The model under review builds one solid part; all positions refer to its coordinate system, in mm. Face numbers are marked on the shaded views. A direction names the side the tool comes from. Round coordinates to 2 decimals unless told otherwise and drop trailing zeros. Order: outer loops, then holes, each group sorted by start corner. A loop starts at its lowest first (then second) coordinate and runs counter-clockwise, first axis right, second up.
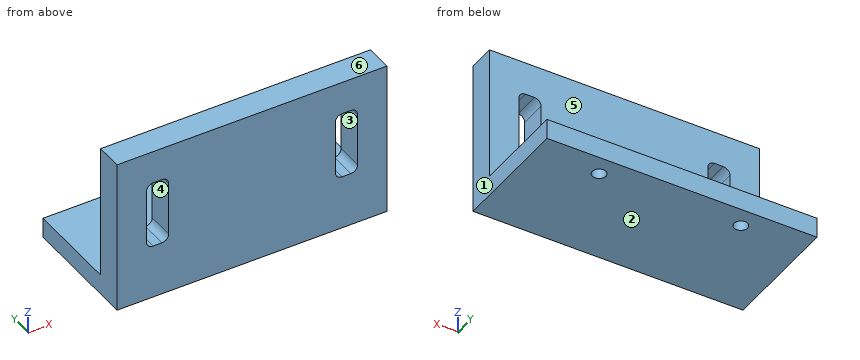
from build123d import *

# Parameters (mm, degrees)
SKETCH1_W           = 40
SKETCH1_H           = 20
BOSS_EXTRUDE1_DEPTH = 4
SKETCH2_W           = 40
SKETCH2_H           = 3
BOSS_EXTRUDE2_DEPTH = 18
SKETCH3_R           = 1
CUT_EXTRUDE1_DEPTH  = 36.397740041


with BuildPart() as part:
    # Sketch1 → Boss-Extrude1 (new body)
    with BuildSketch(Plane(origin=(0, 0, 0), x_dir=(1, 0, 0), z_dir=(0, 1, 0))):
        Rectangle(SKETCH1_W, SKETCH1_H)
        with BuildLine():
            Line((13.35, 4.93188921), (14.65, 4.93188921))
            ThreePointArc((14.65, 4.93188921), (15.357106781, 4.638995992), (15.65, 3.93188921))
            Line((15.65, 3.93188921), (15.65, -4.06811079))
            ThreePointArc((15.65, -4.06811079), (15.357106781, -4.775217571), (14.65, -5.06811079))
            Line((14.65, -5.06811079), (13.35, -5.06811079))
            ThreePointArc((13.35, -5.06811079), (12.642893219, -4.775217571), (12.35, -4.06811079))
            Line((12.35, -4.06811079), (12.35, 3.93188921))
            ThreePointArc((12.35, 3.93188921), (12.642893219, 4.638995992), (13.35, 4.93188921))
        make_face(mode=Mode.SUBTRACT)
        with BuildLine():
            Line((-15.65, 3.93188921), (-15.65, -4.06811079))
            ThreePointArc((-15.65, -4.06811079), (-15.357106781, -4.775217571), (-14.65, -5.06811079))
            Line((-14.65, -5.06811079), (-13.35, -5.06811079))
            ThreePointArc((-13.35, -5.06811079), (-12.642893219, -4.775217571), (-12.35, -4.06811079))
            Line((-12.35, -4.06811079), (-12.35, 3.93188921))
            ThreePointArc((-12.35, 3.93188921), (-12.642893219, 4.638995992), (-13.35, 4.93188921))
            Line((-13.35, 4.93188921), (-14.65, 4.93188921))
            ThreePointArc((-14.65, 4.93188921), (-15.357106781, 4.638995992), (-15.65, 3.93188921))
        make_face(mode=Mode.SUBTRACT)
    extrude(amount=BOSS_EXTRUDE1_DEPTH)

    # Sketch2 → Boss-Extrude2 (add)
    with BuildSketch(Plane(origin=(0, 0, 0), x_dir=(1, 0, 0), z_dir=(0, 1, 0))):
        with Locations((0, 11.5)):
            Rectangle(SKETCH2_W, SKETCH2_H)
    extrude(amount=BOSS_EXTRUDE2_DEPTH)

    # Sketch3 → Cut-Extrude1 (cut, through all)
    with BuildSketch(Plane(origin=(0, 0, -13), x_dir=(-1, 0, 0), z_dir=(0, 0, -1))):
        with Locations((10.5, 15.063230043)):
            Circle(SKETCH3_R)
        with Locations((-10.5, 15.063230043)):
            Circle(SKETCH3_R)
    extrude(amount=-CUT_EXTRUDE1_DEPTH, mode=Mode.SUBTRACT)


solid = part.part
(1) We need section A-A (z = 2.75). Give the boundary of the cut face in (x, y), and give its area (3 significant figures).
(2) We need section C-C (y = 1.5). Give the boundary of the cut face in (x, z).
(3) To check wall thickness, follow L1, parallel to X at y = 1, z = 3.75; L2, parallel to Y at x = -10.5, z = -10.95; L3, parallel to Y at x = 0, z = -6. State the ranges of each line that lie inside material, in increasing order.
(4) We need section D-D (x = 5). Give the boundary of the cut face in (y, z).
(5) We need section B-B (x = 10.5). Give the boundary of the cut face in (y, z), and give its area (3 significant figures).
(6) The part is to be moulded in two halves that separate along X. For the marked faces 1, 2 and 3, say which applies: pulls with the +X half, pulls with the -X half, needs draft (parallel to the pull), parting line crosses it, or undercut.
(7) Tool access review of the marked faces 4, 5 and 6: name each direction out of +Z, -Z, +X, -X, +Y, -Y from which nothing blocks a thin tool from reaching the whole face with its end or side.
(8) Clearance check with flat-ended pins moving along their axes: P1, Ø2, axis at x = 11.5, y = 15, coming from the +Z side; P2, Ø1.8, axis at x = -10.5, y = 15.06, coming from the -Z side; P3, Ø1, axis at x = 15.5, z = 6.5, coming from the +Y side. State where each tip first meets the part, or that it passes through.
Verdict:
1. outline: (-20, 0) - (-15.65, 0) - (-15.65, 4) - (-20, 4) - close; (-12.35, 0) - (12.35, 0) - (12.35, 4) - (-12.35, 4) - close; (15.65, 0) - (20, 0) - (20, 4) - (15.65, 4) - close
1. area: 134 mm2
2. outline: (-20, -13) - (20, -13) - (20, 10) - (-20, 10) - close; hole (-15.65, -3.93) arc R1 ccw to (-14.65, -4.93) - (-13.35, -4.93) arc R1 ccw to (-12.35, -3.93) - (-12.35, 4.07) arc R1 ccw to (-13.35, 5.07) - (-14.65, 5.07) arc R1 ccw to (-15.65, 4.07) - close; hole (12.35, -3.93) arc R1 ccw to (13.35, -4.93) - (14.65, -4.93) arc R1 ccw to (15.65, -3.93) - (15.65, 4.07) arc R1 ccw to (14.65, 5.07) - (13.35, 5.07) arc R1 ccw to (12.35, 4.07) - close
3. L1: x = -20 to -15.65, -12.35 to 12.35, 15.65 to 20
3. L2: y = 0 to 14.06, 16.06 to 18
3. L3: y = 0 to 4
4. outline: (0, -13) - (18, -13) - (18, -10) - (4, -10) - (4, 10) - (0, 10) - close
5. outline: (0, -13) - (14.06, -13) - (14.06, -10) - (4, -10) - (4, 10) - (0, 10) - close; (16.06, -13) - (18, -13) - (18, -10) - (16.06, -10) - close
5. area: 128 mm2
6. face 1: pulls with the +X half
6. face 2: needs draft
6. face 3: undercut
7. face 4: +Y, -Y
7. face 5: +Z, +X, -X, +Y
7. face 6: +Z, +X, -X, +Y, -Y
8. P1: stops at z = -10
8. P2: passes through
8. P3: stops at y = 4
